from build123d import *

# Parameters (mm, degrees)
SKETCH1_W           = 2.5
SKETCH1_H           = 1
BOSS_EXTRUDE1_DEPTH = 1
SKETCH1_4_W         = 2.5
SKETCH1_4_H         = 1
BOSS_EXTRUDE3_DEPTH = 1


with BuildPart() as part:
    # Sketch1 → Boss-Extrude1 (new body)
    with BuildSketch(Plane(origin=(0, 0, 0), x_dir=(1, 0, 0), z_dir=(0, 1, 0))):
        Polygon((5, 9), (5, 10), (0, 10), (0, 0), (5, 0), (5, 1), (1, 1), (1, 9), align=None)
        with BuildLine():
            Line((5, 7.035533906), (5, 9))
            Line((5, 9), (1, 9))
            Line((1, 9), (1, 1))
            Line((1, 1), (5, 1))
            Line((5, 1), (5, 2.964466094))
            ThreePointArc((5, 2.964466094), (2.964466094, 5), (5, 7.035533906))
        make_face()
        with BuildLine():
            ThreePointArc((6.439339828, 6.439339828), (5.778965102, 6.880588113), (5, 7.035533906))
            Line((5, 7.035533906), (5, 6.5))
            ThreePointArc((5, 6.5), (6.060660172, 6.060660172), (6.5, 5))
            ThreePointArc((6.5, 5), (6.060660172, 3.939339828), (5, 3.5))
            Line((5, 3.5), (5, 2.964466094))
            ThreePointArc((5, 2.964466094), (6.439339828, 3.560660172), (7.035533906, 5))
            ThreePointArc((7.035533906, 5), (6.880588113, 5.778965102), (6.439339828, 6.439339828))
        make_face()
        with BuildLine():
            Line((5, 6.5), (5, 7.035533906))
            ThreePointArc((5, 7.035533906), (2.964466094, 5), (5, 2.964466094))
            Line((5, 2.964466094), (5, 3.5))
            ThreePointArc((5, 3.5), (3.5, 5), (5, 6.5))
        make_face()
        with BuildLine():
            ThreePointArc((6.5, 5), (6.060660172, 6.060660172), (5, 6.5))
            Line((5, 6.5), (5, 3.5))
            ThreePointArc((5, 3.5), (6.060660172, 3.939339828), (6.5, 5))
        make_face()
        with BuildLine():
            Line((5, 3.5), (5, 6.5))
            ThreePointArc((5, 6.5), (3.5, 5), (5, 3.5))
        make_face()
        with BuildLine():
            Line((7.5, 9), (5, 9))
            Line((5, 9), (5, 7.035533906))
            ThreePointArc((5, 7.035533906), (5.778965102, 6.880588113), (6.439339828, 6.439339828))
            ThreePointArc((6.439339828, 6.439339828), (6.114180701, 8.074025149), (7.5, 9))
        make_face()
        with Locations((6.25, 9.5)):
            Rectangle(SKETCH1_W, SKETCH1_H)
        Polygon((10, 10), (7.5, 10), (7.5, 9), (9, 9), (9, 7.5), (10, 7.5), align=None)
        with BuildLine():
            Line((9, 9), (7.5, 9))
            ThreePointArc((7.5, 9), (8.560660172, 8.560660172), (9, 7.5))
            Line((9, 7.5), (9, 9))
        make_face()
        with BuildLine():
            ThreePointArc((9, 7.5), (8.560660172, 8.560660172), (7.5, 9))
            Line((7.5, 9), (7.5, 7.5))
            Line((7.5, 7.5), (9, 7.5))
        make_face()
        with BuildLine():
            Line((7.5, 7.5), (7.5, 9))
            ThreePointArc((7.5, 9), (6.114180701, 8.074025149), (6.439339828, 6.439339828))
            ThreePointArc((6.439339828, 6.439339828), (8.074025149, 6.114180701), (9, 7.5))
            Line((9, 7.5), (7.5, 7.5))
        make_face()
        with BuildLine():
            ThreePointArc((9, 7.5), (8.074025149, 6.114180701), (6.439339828, 6.439339828))
            ThreePointArc((6.439339828, 6.439339828), (6.880588113, 5.778965102), (7.035533906, 5))
            ThreePointArc((7.035533906, 5), (6.439339828, 3.560660172), (5, 2.964466094))
            Line((5, 2.964466094), (5, 1))
            Line((5, 1), (9, 1))
            Line((9, 1), (9, 7.5))
        make_face()
        Polygon((10, 7.5), (9, 7.5), (9, 1), (5, 1), (5, 0), (10, 0), align=None)
    extrude(amount=BOSS_EXTRUDE1_DEPTH)

    # Sketch1_4 → Boss-Extrude3 (add)
    with BuildSketch(Plane(origin=(0, 0, 0), x_dir=(1, 0, 0), z_dir=(0, 1, 0))):
        with BuildLine():
            ThreePointArc((6.439339828, 6.439339828), (5.778965102, 6.880588113), (5, 7.035533906))
            Line((5, 7.035533906), (5, 6.5))
            ThreePointArc((5, 6.5), (6.060660172, 6.060660172), (6.5, 5))
            ThreePointArc((6.5, 5), (6.060660172, 3.939339828), (5, 3.5))
            Line((5, 3.5), (5, 2.964466094))
            ThreePointArc((5, 2.964466094), (6.439339828, 3.560660172), (7.035533906, 5))
            ThreePointArc((7.035533906, 5), (6.880588113, 5.778965102), (6.439339828, 6.439339828))
        make_face()
        with BuildLine():
            Line((5, 6.5), (5, 7.035533906))
            ThreePointArc((5, 7.035533906), (2.964466094, 5), (5, 2.964466094))
            Line((5, 2.964466094), (5, 3.5))
            ThreePointArc((5, 3.5), (3.5, 5), (5, 6.5))
        make_face()
        Polygon((5, 9), (5, 10), (0, 10), (0, 0), (5, 0), (5, 1), (1, 1), (1, 9), align=None)
        Polygon((10, 7.5), (9, 7.5), (9, 1), (5, 1), (5, 0), (10, 0), align=None)
        Polygon((10, 10), (7.5, 10), (7.5, 9), (9, 9), (9, 7.5), (10, 7.5), align=None)
        with Locations((6.25, 9.5)):
            Rectangle(SKETCH1_4_W, SKETCH1_4_H)
    extrude(amount=-BOSS_EXTRUDE3_DEPTH)


solid = part.part
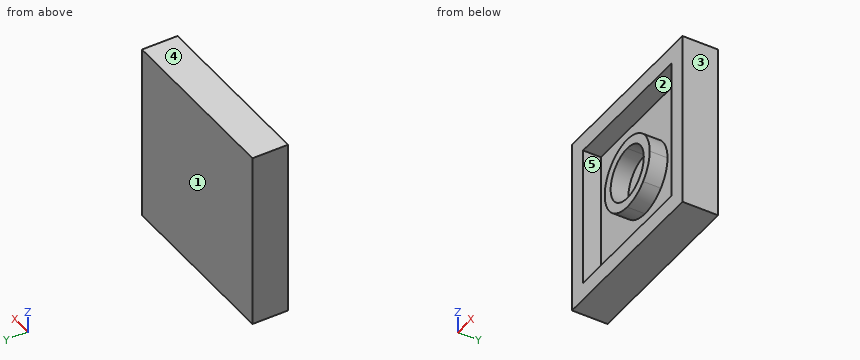
Input: part model. Units: mm. Frame: model coordinates. Face numbers are marked on the shaded views. A direction names the side the tool comes from. Coordinates: 2 decimals unless noted, no trailing zeros. Order: outer loops, then holes, each group sorted by start corner. A loop starts at its lowest first (then second) coordinate and runs counter-clockwise, first axis right, second up. Notation, with made-up numbers: M 65,-31.5 L 74,-31.5 A8 ccw 74,-19.5 Z; hole C 83,13 d4. An arc over 180 degrees is marked long. Answer as CSV lines item,"result".
1. Section D-D (z = -5.5). Return the cut outline in (x, y), then the cut area to 3 significant figures.
Reported:
outline,"M 0,-1 L 1,-1 L 1,0 L 3.03,0 L 3.03,-1 L 3.59,-1 L 3.59,0 L 6.41,0 L 6.41,-1 L 6.97,-1 L 6.97,0 L 9,0 L 9,-1 L 10,-1 L 10,1 L 0,1 Z"
area,"13.1 mm2"
2. Section A-A (y = -0.15). Return the cut outline in (x, z), then the cut area to 3 significant figures.
Reported:
outline,"M 0,-10 L 10,-10 L 10,0 L 0,0 Z; C 5,-5 d4.07; hole M 1,-9 L 9,-9 L 9,-1 L 1,-1 Z; hole C 5,-5 d3"
area,"41.9 mm2"
3. Section B-B (z = -7.5). Return the cut outline in (x, y), then the cut area to 3 significant figures.
Reported:
outline,"M 0,-1 L 1,-1 L 1,0 L 9,0 L 9,-1 L 10,-1 L 10,1 L 0,1 Z"
area,"12.0 mm2"
4. Access query for the marked faces 1 and 2. Directions: +Z, -Z, +X, -X, +Y, -Y. A direction counts if a zero-diameter tool reaches every point of the face in a straight line with its end or side. Return the directions, or none.
Reported:
face 1,"+Z, -Z, +X, -X, +Y"
face 2,"-Y"
5. Section C-C (x = 7.25). Return the cut outline in (y, z).
Reported:
outline,"M -1,-10 L 1,-10 L 1,0 L -1,0 L -1,-1 L 0,-1 L 0,-9 L -1,-9 Z"
6. Material intervals for line 1 (Z direction, x = 1.25, y = -0.55); line 2 (X direction, y = -0.15, z = -4.5); line 3 (X direction, y = -0.1, z = -1.25), sorted ascending. Write a range as from..to.
Reported:
line 1,"-10..-9, -1..0"
line 2,"0..1, 3.03..3.59, 6.41..6.97, 9..10"
line 3,"0..1, 9..10"
7. Pull-direction query (Z, two-part tool) for the marked faces 3, 4 and 5; classes: released by +Z, released by -Z, zero draft, split by the parting line, or undercut.
Reported:
face 3,"zero draft"
face 4,"released by +Z"
face 5,"undercut"
